Autodesk Inventor part; units mm, degrees
ref_plane "YZ Plane" through (0, 0, 0) normal (1, 0, 0) x (0, 1, 0)
ref_plane "XZ Plane" through (0, 0, 0) normal (0, 1, 0) x (-1, 0, 0)
ref_plane "XY Plane" through (0, 0, 0) normal (0, 0, 1) x (1, 0, 0)
sketch "Эскиз1" plane through (0, 0, 0) normal (0, 1, 0) x (-1, 0, 0)
  arc A0 (0, -5.25) -> (0, 5.25) centre (0, 0) ccw
  arc A1 (0, -7.5) -> (0, 7.5) centre (0, 0) ccw
  line L0 (0, 7.5) -> (-0.25, 7.5)
  line L1 (-5.25, 6.25) -> (-5.25, 17.5)
  line L2 (-5.25, -17.5) -> (-5.25, -6.25)
  line L3 (-0.25, -7.5) -> (0, -7.5)
  line L4 (-5.25, 17.5) -> (-2.25, 17.5)
  line L5 (-2.25, 17.5) -> (-2.25, 9.5)
  line L6 (-2.25, -9.5) -> (-2.25, -17.5)
  line L7 (-2.25, -17.5) -> (-5.25, -17.5)
  line L8 (0, 5.25) -> (-4.25, 5.25)
  line L9 (0, -5.25) -> (-4.25, -5.25)
  arc A2 (-2.25, 9.5) -> (-0.25, 7.5) centre (-0.25, 9.5) ccw
  arc A3 (-0.25, -7.5) -> (-2.25, -9.5) centre (-0.25, -9.5) ccw
  arc A4 (-5.25, 6.25) -> (-4.25, 5.25) centre (-4.25, 6.25) ccw
  arc A5 (-4.25, -5.25) -> (-5.25, -6.25) centre (-4.25, -6.25) ccw
  point P0 (-2.25, -7.5)
  dimension "d0" = 10.5
  dimension "d4" = 3
  dimension "d5" = 2
  dimension "d6" = 1
extrude "Выдавливание1" add sketch "Эскиз1" along normal blind 12
fillet "Сопряжение1" radius 5 4 edges at (3.75, 12, 17.5) (3.75, 0, 17.5) (3.75, 12, -17.5) (3.75, 0, -17.5)
sketch "Эскиз2" plane through (2.25, 0, 9.5) normal (-1, 0, 0) x (0, 0, 1)
  line L0 (8, 5) -> (8, 7)
  line L1 (8, 6) -> (3, 6)
  circle A0 centre (3, 6) radius 1.75
  line L2 (-27, 5) -> (-27, 7)
  line L3 (-27, 6) -> (-22, 6)
  circle A1 centre (-22, 6) radius 1.75
  point P0 (-9.5, 0)
  dimension "d10" = 5
  dimension "d11" = 3.5
  dimension "d12" = 5
  dimension "d13" = 3.5
extrude "Выдавливание2" cut sketch "Эскиз2" against normal through all
fillet "Сопряжение2" radius 0.6 20 edges at (0.125, 12, 7.5) (1.6642, 12, 8.0858) (2.25, 12, 11) (2.25, 10.5355, 16.0355) (2.25, 6, 17.5) (2.25, 1.4645, 16.0355) (2.25, 0, 11) (1.6642, 0, 8.0858) (0.125, 0, 7.5) (-7.5, 0, 0) (0.125, 0, -7.5) (1.6642, 0, -8.0858) (2.25, 0, -11) (2.25, 1.4645, -16.0355) (2.25, 6, -17.5) (2.25, 10.5355, -16.0355) (2.25, 12, -11) (1.6642, 12, -8.0858) (0.125, 12, -7.5) (-7.5, 12, 0)
properties part number "tube_holder"
Can you work these out from the model? Positions are in its coordinate system, mm. A direction names the side the tool comes from. Round coordinates to 2 decimals unless told otherwise and drop trailing zeros. Write each loop counter-clockwise with the first axis right and the second up, starting at its lowest first coordinate (ties: lowest second). Pieces come first, ordered by that corner, then holes. Notation, with made-up numbers: M -9.5,9 L 35.5,9 A18 cw 35.5,36 Z; hole C 47.5,-5 d4. An arc over 180 degrees is marked long. Use a Markdown table: item, result.
Item 1: If I drill on line 1 along Y through (x, z) = (4.65, 12.5); line 2 along Z through (x, y) = (-3.5, 9.25); line 3 along Z through (x, y) = (0.25, 5.25), over which ranges is the centre line in solid material (lowest first)? Write a range as [from, to].
Found:
| item | result |
|---|---|
| line 1 | y = [0, 4.25], [7.75, 12] |
| line 2 | z = [-6.63, -3.91], [3.91, 6.63] |
| line 3 | z = [-7.5, -5.25], [5.25, 7.5] |
Item 2: We'd pull the mould along Z, two halves only. Please class faces 4 (the face through (4.07, 10.5, -16.07)), 5 (the face through (5.25, 4.6, -10.7)), 6 (the face through (2, 6, 5.25)): released by +Z, released by -Z, zero draft, split by the parting line, or undercut.
Found:
| item | result |
|---|---|
| face 4 | released by -Z |
| face 5 | zero draft |
| face 6 | undercut |
Item 3: I want a section at C-C (z = 0). List the corners of the cut face in (x, y) for me.
Found:
| item | result |
|---|---|
| outline | M -7.5,0.6 A0.6 ccw -6.9,0 L -5.25,0 L -5.25,12 L -6.9,12 A0.6 ccw -7.5,11.4 Z |
Item 4: I want a section at A-A (x = 3.75). List the corners of the cut face in (y, z) for me, and give its area (3 significant figures).
Found:
| item | result |
|---|---|
| outline | M 0,-12.5 A5 ccw 5,-17.5 L 7,-17.5 A5 ccw 12,-12.5 L 12,-5.25 L 0,-5.25 Z; M 0,5.25 L 12,5.25 L 12,12.5 A5 ccw 7,17.5 L 5,17.5 A5 ccw 0,12.5 Z; hole C 6,-12.5 d3.5; hole C 6,12.5 d3.5 |
| area | 253 mm2 |
Item 5: I want a section at B-B (y = 6). List the corners of the cut face in (x, z) for me.
Found:
| item | result |
|---|---|
| outline | M 0,-7.5 L 0.25,-7.5 A2 cw 2.25,-9.5 L 2.25,-10.75 L 5.25,-10.75 L 5.25,-6.25 A1 ccw 4.25,-5.25 L 0,-5.25 A5.25 cw 0,5.25 L 4.25,5.25 A1 ccw 5.25,6.25 L 5.25,10.75 L 2.25,10.75 L 2.25,9.5 A2 cw 0.25,7.5 L 0,7.5 A7.5 ccw Z; M 2.25,-16.9 A0.6 ccw 2.85,-17.5 L 5.25,-17.5 L 5.25,-14.25 L 2.25,-14.25 Z; M 2.25,14.25 L 5.25,14.25 L 5.25,17.5 L 2.85,17.5 A0.6 ccw 2.25,16.9 Z |
Item 6: For pin 1 Ø4 at (y, z) = (6, -12.5) entering from +X; pin 2 Ø2 at (y, z) = (3.5, 11.5) entering from -X; pin 3 Ø2 at (x, y) = (-4, 3.5) entering from +Z; pin 4 Ø1.5 at (x, y) = (2.5, 2.5) entering from +Z, each with a flat end and sliding along its axis, tell me the tip position at first contact or that it passes through.
Found:
| item | result |
|---|---|
| pin 1 | stops at x = 5.25 |
| pin 2 | stops at x = 2.25 |
| pin 3 | stops at z = 6.87 |
| pin 4 | stops at z = 17.16 |
Item 7: Which directions (+Z, -Z, +X, -X, +Y, -Y) give clear straight access to the entire face, cutting with the end or side of a thin tool? Please do faces 1 (the face through (2, 6, -5.25)), 2 (the face through (2.25, 7.1, 14.1)), 3 (the face through (2.25, 4.7, -14)).
Found:
| item | result |
|---|---|
| face 1 | +X, +Y, -Y |
| face 2 | +Z, -X, +Y, -Y |
| face 3 | -Z, -X, +Y, -Y |
